Design review of the part built by this model. Coordinates are the model's own, in mm. Round coordinates to 2 decimals unless told otherwise and drop trailing zeros. Order: outer loops, then holes, each group sorted by start corner. A loop starts at its lowest first (then second) coordinate and runs counter-clockwise, first axis right, second up. Notation, with made-up numbers: (-8.5, 25.25) - (31.5, 25.25) arc R14 cw to (31.5, 35.25) - close; hole circle Ø4 at (-15, 47). An arc over 180 degrees is marked (long way). Use CSV: the item, a comma, the result in double quotes.
Autodesk Inventor part; units mm, degrees
ref_plane "YZ Plane" through (0, 0, 0) normal (1, 0, 0) x (0, 1, 0)
ref_plane "XZ Plane" through (0, 0, 0) normal (0, 1, 0) x (-1, 0, 0)
ref_plane "XY Plane" through (0, 0, 0) normal (0, 0, 1) x (1, 0, 0)
sketch "Sketch1" plane through (0, 0, 0) normal (0, 0, 1) x (1, 0, 0)
  line L0 (-207, 22.5) -> (207, 22.5)
  line L1 (207, 22.5) -> (207, -22.5)
  line L2 (207, -22.5) -> (-207, -22.5)
  line L3 (-207, -22.5) -> (-207, 22.5)
  line L4 (-207, 22.5) -> (207, -22.5) construction
  line L5 (207, 22.5) -> (-207, -22.5) construction
  point P0 (0, 0)
  dimension "d0" = 414
  dimension "d1" = 45
extrude "Extrusion1" add sketch "Sketch1" along normal mid plane 3
sketch "Sketch2" plane through (0, 0, 1.5) normal (0, 0, 1) x (1, 0, 0)
  line L0 (-207, 22.5) -> (-207, -22.5)
  line L1 (207, -22.5) -> (207, 22.5)
  line L2 (-207, -22.5) -> (207, -22.5)
  point P0 (0, 0)
  point P1 (-182, -8.5)
  point P2 (0, -8.5)
  point P3 (182, -8.5)
  dimension "d4" = 25
  dimension "d5" = 25
  dimension "d6" = 182
  dimension "d7" = 14
hole "Hole1" at (-182, -8.5, 1.5) at (0, -8.5, 1.5) at (182, -8.5, 1.5) direction (0, 0, -1) diameter 6 depth 14.2 tip angle 118
sketch "Sketch3" plane through (0, 0, 1.5) normal (0, 0, 1) x (1, 0, 0)
  line L0 (-207, 22.5) -> (207, 22.5)
  line L1 (-148, 22.5) -> (-123, 22.5)
  line L2 (-123, 22.5) -> (-123, 12.5)
  line L3 (-123, 12.5) -> (-148, 12.5)
  line L4 (-148, 12.5) -> (-148, 22.5)
  line L5 (207, -22.5) -> (207, 22.5)
  point P0 (0, 0)
  point P1 (-123, 22.5)
  dimension "d15" = 330
  dimension "d16" = 25
  dimension "d17" = 10
extrude "Extrusion2" cut sketch "Sketch3" against normal blind 3
sketch "Sketch5" plane through (0, 0, 1.5) normal (0, 0, 1) x (1, 0, 0)
  line L0 (-148, 22.5) -> (-207, 22.5)
  line L1 (-207, 22.5) -> (137, 22.5)
  line L2 (137, 22.5) -> (137, 32.5)
  line L3 (137, 32.5) -> (-207, 32.5)
  line L4 (-207, 32.5) -> (-207, 22.5)
  line L5 (207, -22.5) -> (207, 22.5)
  line L6 (-148, 22.5) -> (-148, 32.5)
  line L7 (-123, 22.5) -> (207, 22.5)
  line L8 (-123, 22.5) -> (-123, 32.5)
  point P0 (0, 0)
  dimension "d23" = 70
  dimension "d24" = 10
extrude "Extrusion4" add sketch "Sketch5" against normal blind 3 contours L0 L4 L3 L6 | L8 L3 L2 L1
properties part number "HCMUTE-CDT23-KXL_A01" material "PMMA Plastic"
1) We need section A-A (y = 26.5). Give the boundary of the cut face in (x, z), then the cut area to 3 significant figures.
Data:
outline,"(-207, -1.5) - (-148, -1.5) - (-148, 1.5) - (-207, 1.5) - close; (-123, -1.5) - (137, -1.5) - (137, 1.5) - (-123, 1.5) - close"
area,"957 mm2"
2) To check wall thickness, follow L1, parallel to X at y = -8.5, z = -0.05; L2, parallel to X at y = 29.5, z = -1.25; L3, parallel to Y at x = 0, z = 0.1. State the ranges of each line that lie inside material, in increasing order. Write a range as from..to.
Data:
L1,"x = -207..-185, -179..-3, 3..179, 185..207"
L2,"x = -207..-148, -123..137"
L3,"y = -22.5..-11.5, -5.5..32.5"
3) We need section B-B (z = 0.7). Give the boundary of the cut face in (x, y).
Data:
outline,"(-207, -22.5) - (207, -22.5) - (207, 22.5) - (137, 22.5) - (137, 32.5) - (-123, 32.5) - (-123, 12.5) - (-148, 12.5) - (-148, 32.5) - (-207, 32.5) - close; hole circle Ø6 at (-182, -8.5); hole circle Ø6 at (0, -8.5); hole circle Ø6 at (182, -8.5)"
4) Insertion check: pin 1 Ø3.5 at (x, y) = (0, -8.5) entering from +Z; pin 2 Ø0.9 at (y, z) = (26.5, 0) entering from +X; pin 3 Ø9.5 at (x, y) = (182, -8.5) entering from +Z. Each pin has a flat end and moves straight along its axis. Give the tip position at first contact, or say it passes through.
Data:
pin 1,"passes through"
pin 2,"stops at x = 137"
pin 3,"stops at z = 1.5"
5) We need section D-D (x = 142.5). Give the boundary of the cut face in (y, z), then the cut area to 3 significant figures.
Data:
outline,"(-22.5, -1.5) - (22.5, -1.5) - (22.5, 1.5) - (-22.5, 1.5) - close"
area,"135 mm2"
6) We need section C-C (x = -142.5). Give the boundary of the cut face in (y, z).
Data:
outline,"(-22.5, -1.5) - (12.5, -1.5) - (12.5, 1.5) - (-22.5, 1.5) - close"
